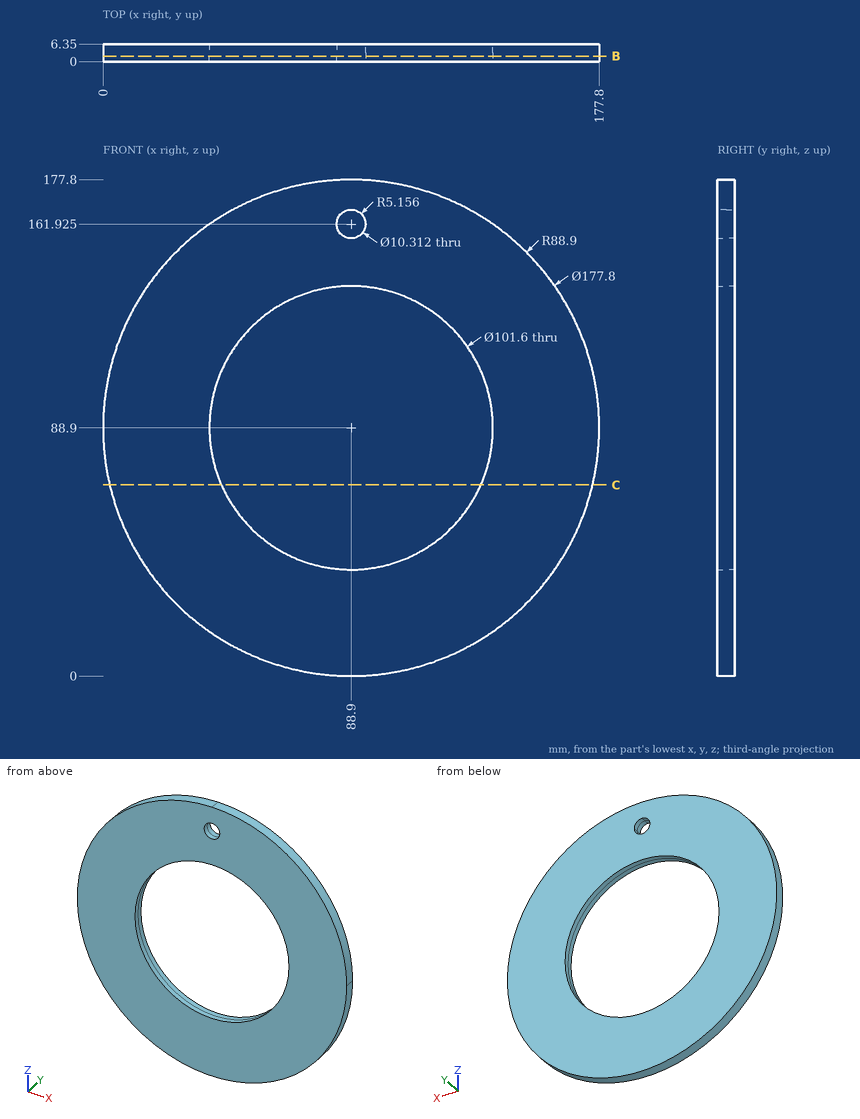
Drawing for the job (mm, zero at the part's lowest x, y, z). Give positions to 0.01 mm unless a question says otherwise; leave off trailing zeros. Order: outer loops, then holes, each group sorted by start corner. A loop starts at its lowest first (then second) coordinate and runs counter-clockwise, first axis right, second up. Notation, with made-up numbers: (-18, -9) - (-8, -9) arc R13 ccw to (-8, 12) - close; hole circle Ø10 at (88, 11.5). An arc over 180 degrees is marked (long way). Write item = value, one per line. Start each with the question number.
1. Cut at C-C, the plane z = 68.5. List the corners of the cut face in (x, y), and give its area (3 significant figures).
2. Probe line 1 along Z through (x, y) = (80, 0.5) (1 decimal); line 2 along X through (y, z) = (3, 129) (1 decimal); line 3 along Z through (x, y) = (88, 3) (1 decimal). List the from-to ranges inside material, lowest first.
3. Drop flat-ended pins along their axis: P1, Ø1, axis at y = 2.5, z = 123.5, coming from the -X side; P2, Ø2, axis at x = 150.5, y = 3, coming from the +Z side (1 decimal); P3, Ø9.5, axis at x = 88.9, z = 161.925, coming from the -Y side; P4, Ø1.5, axis at x = 43.5, y = 1.5, coming from the +Z side. Give the stop position or say it passes through.
4. Cut at B-B, the plane y = 2. List the corners of the cut face in (x, z) (1 decimal).
Taken from the geometry:
q1.outline = (2.37, 0) - (42.38, 0) - (42.38, 6.35) - (2.37, 6.35) - close; (135.42, 0) - (175.43, 0) - (175.43, 6.35) - (135.42, 6.35) - close
q1.area = 508 mm²
q2.line_1 = 0.4 to 38.9, 138.9 to 177.4
q2.line_2 = 9.6 to 57.7, 120.1 to 168.2
q2.line_3 = 0 to 38.1, 139.7 to 156.8, 167 to 177.8
q3.P1 = 6.8
q3.P2 = 153.9
q3.P3 = through
q3.P4 = 165.77
q4.outline = circle Ø177.8 at (88.9, 88.9); hole circle Ø101.6 at (88.9, 88.9); hole circle Ø10.3 at (88.9, 161.9)
